Part model, mm, in its own coordinate system. Face numbers are marked on the shaded views. A direction names the side the tool comes from. Coordinates: 2 decimals unless noted, no trailing zeros. Order: outer loops, then holes, each group sorted by start corner. A loop starts at its lowest first (then second) coordinate and runs counter-clockwise, first axis right, second up.
1) Wall check: L1, parallel to Z at x = 26.5, y = -0.5; L2, parallel to Z at x = 13, y = 3.5; L3, parallel to X at y = 4.5, z = -4.75. Give the ranges that are in metal, low to high.
2) Tool access for the marked faces 1, 2, 3, 4 and 5: list every direction of +Z, -Z, +X, -X, +Y, -Y with a clear straight run to the whole face (end or side of a thin tool).
3) Pin check, flat tips, straight feed: pin 1 Ø3 at (x, z) = (21, -8.5) entering from -Y; pin 2 Ø1.5 at (x, y) = (14.5, 3.5) entering from +Z; pin 3 Ø2 at (x, z) = (24.5, -5.5) entering from +Y. Stop position of each tip, or through.
4) Cut at A-A (x = 26). List the corners of the cut face in (y, z), and give its area (3 significant figures).
5) Cut at C-C (z = -6.5). List the corners of the cut face in (x, y), and give its area (3 significant figures).
6) Cut at D-D (x = 6). List the corners of the cut face in (y, z).
7) Cut at B-B (y = 0.5). List the corners of the cut face in (x, z).
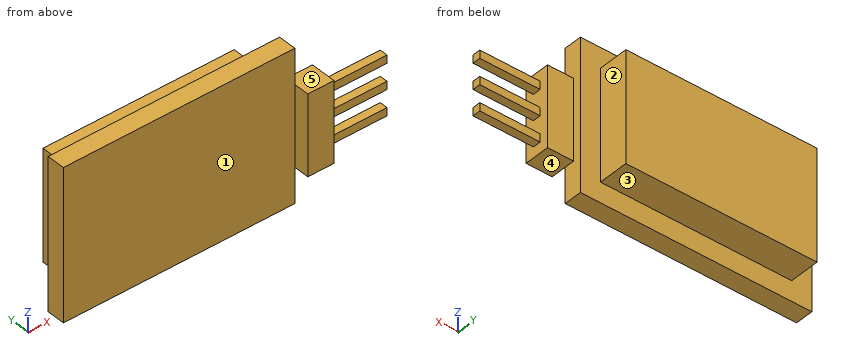
```python
from build123d import *

# Parameters (mm, degrees)
CROQUIS1_W              = 23
CROQUIS1_H              = 15
SALIENTE_EXTRUIR1_DEPTH = 1.8
CROQUIS2_W              = 19
CROQUIS2_H              = 11
SALIENTE_EXTRUIR2_DEPTH = 3
CROQUIS3_W              = 8
CROQUIS3_H              = 2.54
SALIENTE_EXTRUIR3_DEPTH = 2.6
CROQUIS4_W              = 0.8
CROQUIS4_H              = 0.8
SALIENTE_EXTRUIR4_DEPTH = 6


with BuildPart() as part:
    # Croquis1 → Saliente-Extruir1 (new body)
    with BuildSketch(Plane(origin=(0, 0, 0), x_dir=(1, 0, 0), z_dir=(0, 1, 0))):
        with Locations((11.5, 7.5)):
            Rectangle(CROQUIS1_W, CROQUIS1_H)
    extrude(amount=SALIENTE_EXTRUIR1_DEPTH)

    # Croquis2 → Saliente-Extruir2 (add)
    with BuildSketch(Plane(origin=(0, 1.8, 0), x_dir=(1, 0, 0), z_dir=(0, 1, 0))):
        with Locations((11.5, 7.5)):
            Rectangle(CROQUIS2_W, CROQUIS2_H)
    extrude(amount=SALIENTE_EXTRUIR2_DEPTH)

    # Croquis3 → Saliente-Extruir3 (add)
    with BuildSketch(Plane(origin=(23, 0, 0), x_dir=(0, 0, -1), z_dir=(1, 0, 0))):
        with Locations((7.5, -0.27)):
            Rectangle(CROQUIS3_W, CROQUIS3_H)
    extrude(amount=SALIENTE_EXTRUIR3_DEPTH)

    # Croquis4 → Saliente-Extruir4 (add)
    with BuildSketch(Plane(origin=(25.6, 0, 0), x_dir=(0, 0, -1), z_dir=(1, 0, 0))):
        with Locations((10.04, -0.27)):
            Rectangle(CROQUIS4_W, CROQUIS4_H)
        with Locations((7.5, -0.27)):
            Rectangle(CROQUIS4_W, CROQUIS4_H)
        with Locations((4.96, -0.27)):
            Rectangle(CROQUIS4_W, CROQUIS4_H)
    extrude(amount=SALIENTE_EXTRUIR4_DEPTH)


solid = part.part
```
Geometry check:
1. L1: z = -10.44 to -9.64, -7.9 to -7.1, -5.36 to -4.56
1. L2: z = -13 to -2
1. L3: x = 2 to 21
2. face 1: +Z, -Z, -X, -Y
2. face 2: +Z, -Z, +X, +Y
2. face 3: -Z, +X, -X, +Y
2. face 4: -Z, +X, +Y, -Y
2. face 5: +Z, +X, +Y, -Y
3. pin 1: stops at y = 0
3. pin 2: stops at z = -2
3. pin 3: stops at y = 1
4. outline: (-0.67, -10.44) - (0.13, -10.44) - (0.13, -9.64) - (-0.67, -9.64) - close; (-0.67, -7.9) - (0.13, -7.9) - (0.13, -7.1) - (-0.67, -7.1) - close; (-0.67, -5.36) - (0.13, -5.36) - (0.13, -4.56) - (-0.67, -4.56) - close
4. area: 1.92 mm2
5. outline: (0, 0) - (23, 0) - (23, -1.54) - (25.6, -1.54) - (25.6, 1) - (23, 1) - (23, 1.8) - (21, 1.8) - (21, 4.8) - (2, 4.8) - (2, 1.8) - (0, 1.8) - close
5. area: 105 mm2
6. outline: (0, -15) - (1.8, -15) - (1.8, -13) - (4.8, -13) - (4.8, -2) - (1.8, -2) - (1.8, 0) - (0, 0) - close
7. outline: (0, -15) - (23, -15) - (23, -11.5) - (25.6, -11.5) - (25.6, -3.5) - (23, -3.5) - (23, 0) - (0, 0) - close
